```python
from build123d import *

# Parameters (mm, degrees)
SKETCH3_R               = 25.4
BOSS_EXTRUDE1_DEPTH     = 25.4
SKETCH4_R               = 12.7
BOSS_EXTRUDE2_DEPTH     = 12.7
CUT_EXTRUDE1_DEPTH      = 26.4
CUT_EXTRUDE1_DEPTH_BACK = 26.4


with BuildPart() as part:
    # Sketch3 → Boss-Extrude1 (new body)
    with BuildSketch(Plane(origin=(0, 0, 0), x_dir=(1, 0, 0), z_dir=(0, 1, 0))):
        Circle(SKETCH3_R)
    extrude(amount=BOSS_EXTRUDE1_DEPTH)

    # Sketch4 → Boss-Extrude2 (add)
    with BuildSketch(Plane(origin=(0, 25.4, 0), x_dir=(1, 0, 0), z_dir=(0, 1, 0))):
        Circle(SKETCH4_R)
    extrude(amount=BOSS_EXTRUDE2_DEPTH)

    # Sketch5 → Cut-Extrude1 (cut, two sides)
    with BuildSketch(Plane(origin=(0, 0, 0), x_dir=(0, 0, -1), z_dir=(1, 0, 0))) as cut_extrude1_sk:
        Polygon((12.7, 6.35), (-12.7, 6.35), (-12.7, 19.05), (0, 19.05), (0, 9.525), (12.7, 9.525), align=None)
    extrude(amount=CUT_EXTRUDE1_DEPTH, mode=Mode.SUBTRACT)
    extrude(cut_extrude1_sk.sketch, amount=-CUT_EXTRUDE1_DEPTH_BACK, mode=Mode.SUBTRACT)


solid = part.part
```
Build history of the part. All positions in model axes, mm. A direction names the side the tool comes from. Round coordinates to 2 decimals unless told otherwise and drop trailing zeros. Loops run counter-clockwise (first coordinate to the right, second up) from the corner with the lowest first, then second, coordinate; pieces in that order, holes last.
Item 1: Two-plate mould, pull along Z, no slides. Class faces 4 (the face through (0, 0, 0)), 5 (the face through (-25.375, 12.522, -1.117)), 6 (the face through (0, 6.35, 0)): released by +Z, released by -Z, zero draft, split by the parting line, or undercut.
Item 2: Which spindle directions (+Z, -Z, +X, -X, +Y, -Y) get a long thin tool onto all of the face, cutting with end or side? Do faces 1 (the face through (5, 25.4, -12)), 2 (the face through (0, 19.05, 6)), 3 (the face through (0, 38.1, 0)). Say none if no direction does.
Item 3: Saw through at A-A (x = 0). List the corners of the cut face in (y, z) (3 decimals).
Item 4: Saw through at C-C (y = 8). List the corners of the cut face in (x, z).
Item 5: Drill centre lines: line 1 along Y through (x, z) = (-15.5, -3) (3 decimals); line 2 along Y through (x, z) = (-12, 10); line 3 along Y through (x, z) = (-0.5, 20). Where is each one in solid material? Low to high.
Item 6: Pin check, flat tips, straight feed: P1, Ø12, axis at x = -12.5, y = 19, coming from the -Z side; P2, Ø6, axis at x = 1, y = 13, coming from the -Z side; P3, Ø1, axis at x = -9.5, y = 8, coming from the +Z side; P4, Ø1, axis at x = 7, z = 4.5, coming from the -Y side. Stop position of each tip, or through.
Item 7: Saw through at B-B (z = -3). List the corners of the cut face in (x, y) (3 decimals), then the cut area to 3 significant figures.
Worked answers:
1. face 4: zero draft
1. face 5: split by the parting line
1. face 6: undercut
2. face 1: +Y
2. face 2: +X, -X
2. face 3: +Z, -Z, +X, -X, +Y
3. outline: (0, -25.4) - (25.4, -25.4) - (25.4, -12.7) - (38.1, -12.7) - (38.1, 12.7) - (25.4, 12.7) - (25.4, 25.4) - (0, 25.4) - close; hole (6.35, -12.7) - (9.525, -12.7) - (9.525, 0) - (19.05, 0) - (19.05, 12.7) - (6.35, 12.7) - close
4. outline: (-22, -12.7) arc R25.4 ccw to (22, -12.7) - close; (-22, 12.7) - (22, 12.7) arc R25.4 ccw to start
5. line 1: y = 0 to 6.35, 9.525 to 25.4
5. line 2: y = 0 to 6.35, 19.05 to 25.4
5. line 3: y = 0 to 25.4
6. P1: stops at z = -24.55
6. P2: stops at z = -25.4
6. P3: stops at z = 23.75
6. P4: stops at y = 0
7. outline: (-25.222, 0) - (25.222, 0) - (25.222, 6.35) - (-25.222, 6.35) - close; (-25.222, 9.525) - (25.222, 9.525) - (25.222, 25.4) - (12.341, 25.4) - (12.341, 38.1) - (-12.341, 38.1) - (-12.341, 25.4) - (-25.222, 25.4) - close
7. area: 1,430 mm2
